Source: CAD feature listing. Evaluate the final solid. Frame: model axes, mm. Give positions to 0.01 mm unless a question says otherwise; leave off trailing zeros. Loops run counter-clockwise (first coordinate to the right, second up) from the corner with the lowest first, then second, coordinate; pieces in that order, holes last. Notation, with made-up numbers: (13, 68) -> (49, 68) arc R24 cw to (49, 104) -> close; hole circle Ø11 at (23, 85.25). An arc over 180 degrees is marked (long way). Return JSON: item names as keys, results as strings. Group by question number.
(1) Pin query (flat end, axial travel): pin 1 (5 mm diameter, centred on x = 1, z = 17.5, fed in from -Y); pin 2 (1 mm diameter, centred on x = -23, y = 2.5, fed in from +Z); pin 3 (1.5 mm diameter, centred on x = -11.5, y = 1.5, fed in from -Z). Return the tip coordinate at first contact, or that it passes through.
(2) Cut plane B-B on x = -13. Return loops of the section in (y, z).
(3) Cut plane A-A on z = 0. Return loops of the section in (x, y), then the cut area to 3 significant figures.
(4) Cut plane D-D on z = 15.5. Return loops of the section in (x, y).
(5) Cut plane C-C on y = 3.95. Return loops of the section in (x, z), then the cut area to 3 significant figures.
(6) Ray query, line 1 (Z direction, x = 1, y = 3.85); line 2 (X direction, y = 1.25, z = 28); line 3 (Z direction, x = -11.5, y = 4.6) (3 decimals). Return the intervals inside material, ascending. Write a range as from..to.
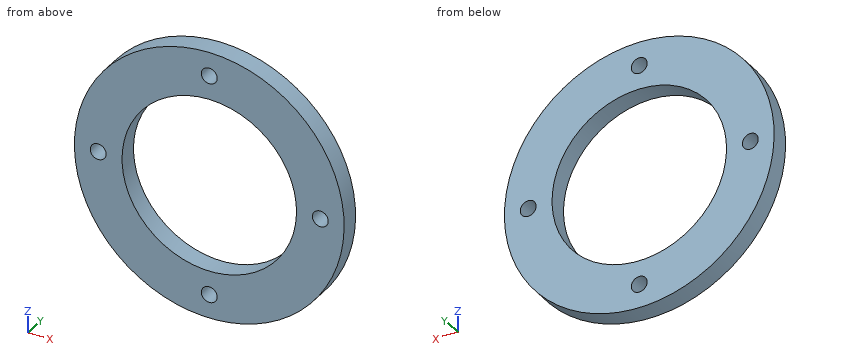
```python
from build123d import *

# Parameters (mm, degrees)
SKETCH_1_R               = 34
EXTRUDE_1_DEPTH          = 5
SKETCH_2_R               = 22
CUT_EXTRUDE_1_DEPTH      = 5
SKETCH_3_R               = 2
CUT_EXTRUDE_2_DEPTH      = 5
PATTERN_CIRCULAR_1_COUNT = 4


with BuildPart() as part:
    # 草图1 → 凸台-拉伸1 (new body)
    with BuildSketch(Plane(origin=(0, 0, 0), x_dir=(1, 0, 0), z_dir=(0, 1, 0))):
        with Locations(Location((0, 0, 0), (0, 0, 270))):
            Circle(SKETCH_1_R)
    extrude(amount=EXTRUDE_1_DEPTH)

    # 草图2 → 切除-拉伸1 (cut)
    with BuildSketch(Plane(origin=(0, 5, 0), x_dir=(1, 0, 0), z_dir=(0, 1, 0))):
        with Locations(Location((0, 0, 0), (0, 0, 270))):
            Circle(SKETCH_2_R)
    extrude(amount=-CUT_EXTRUDE_1_DEPTH, mode=Mode.SUBTRACT)

    # 草图3 → 切除-拉伸2 (cut)
    with BuildSketch(Plane(origin=(0, 5, 0), x_dir=(1, 0, 0), z_dir=(0, 1, 0))):
        with Locations(Location((0, 28, 0), (0, 0, 270))):
            Circle(SKETCH_3_R)
    cut_extrude_2 = extrude(amount=-CUT_EXTRUDE_2_DEPTH, mode=Mode.SUBTRACT)

    # 阵列(圆周)1: 切除-拉伸2 ×4 about axis
    pattern_circular_1_axis = Axis((0, 0, 0), (0, 1, 0))
    for i in range(1, PATTERN_CIRCULAR_1_COUNT):
        add(cut_extrude_2.rotate(pattern_circular_1_axis, i * 360 / PATTERN_CIRCULAR_1_COUNT), mode=Mode.SUBTRACT)


solid = part.part
```
Answers:
{
 "1": {"pin 1": "through", "pin 2": "z = 25.49", "pin 3": "z = -32.26"},
 "2": {"outline": "(0, -31.42) -> (5, -31.42) -> (5, -17.75) -> (0, -17.75) -> close; (0, 17.75) -> (5, 17.75) -> (5, 31.42) -> (0, 31.42) -> close"},
 "3": {"outline": "(-34, 0) -> (-30, 0) -> (-30, 5) -> (-34, 5) -> close; (-26, 0) -> (-22, 0) -> (-22, 5) -> (-26, 5) -> close; (22, 0) -> (26, 0) -> (26, 5) -> (22, 5) -> close; (30, 0) -> (34, 0) -> (34, 5) -> (30, 5) -> close", "area": "80.0 mm²"},
 "4": {"outline": "(-30.26, 0) -> (-15.61, 0) -> (-15.61, 5) -> (-30.26, 5) -> close; (15.61, 0) -> (30.26, 0) -> (30.26, 5) -> (15.61, 5) -> close"},
 "5": {"outline": "circle Ø68 at (0, 0); hole circle Ø4 at (-28, 0); hole circle Ø44 at (0, 0); hole circle Ø4 at (0, -28); hole circle Ø4 at (0, 28); hole circle Ø4 at (28, 0)", "area": "2,060 mm²"},
 "6": {"line 1": "-33.99..-29.73, -26.27..-21.98, 21.98..26.27, 29.73..33.99", "line 2": "-19.29..-2, 2..19.29", "line 3": "-31.996..-18.755, 18.755..31.996"}
}
